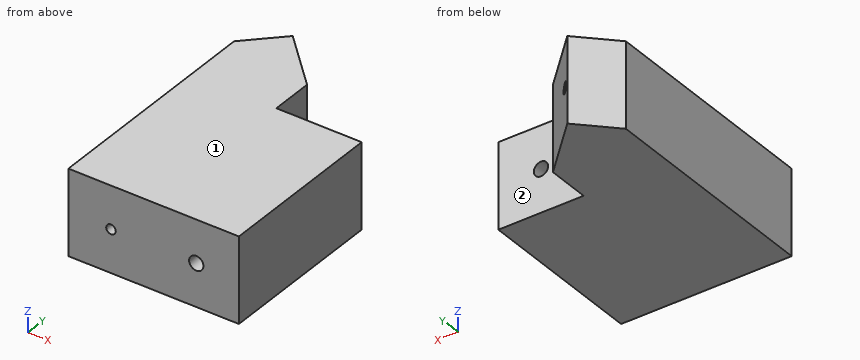
```python
from build123d import *

# Parameters (mm, degrees)
SKETCH1_W               = 10
SKETCH1_H               = 5
BOSS_EXTRUDE1_DEPTH     = 20
SKETCH2_R               = 0.42
SKETCH2_R_2             = 0.28
CUT_EXTRUDE1_DEPTH      = 21
CUT_EXTRUDE2_DEPTH      = 3.5
CUT_EXTRUDE2_DEPTH_BACK = 3.5
CHAMFER1_SIZE2          = 2.828427125
CHAMFER1_SIZE           = 4


with BuildPart() as part:
    # Sketch1 → Boss-Extrude1 (new body)
    with BuildSketch(Plane(origin=(0, 0, 0), x_dir=(1, 0, 0), z_dir=(0, 1, 0))):
        Rectangle(SKETCH1_W, SKETCH1_H)
    extrude(amount=BOSS_EXTRUDE1_DEPTH)

    # Sketch2 → Cut-Extrude1 (cut, through all)
    with BuildSketch(Plane.XZ):
        with Locations((2.5, 0)):
            Circle(SKETCH2_R)
        with Locations((-2.5, 0)):
            Circle(SKETCH2_R_2)
    extrude(amount=-CUT_EXTRUDE1_DEPTH, mode=Mode.SUBTRACT)

    # Sketch3 → Cut-Extrude2 (cut, two sides)
    with BuildSketch(Plane.XY) as cut_extrude2_sk:
        Polygon((-5, 17.5), (0, 12.5), (0, 10), (5, 10), (5, 20), (-5, 20), align=None)
    extrude(amount=CUT_EXTRUDE2_DEPTH, mode=Mode.SUBTRACT)
    extrude(cut_extrude2_sk.sketch, amount=-CUT_EXTRUDE2_DEPTH_BACK, mode=Mode.SUBTRACT)

    # Chamfer1
    chamfer1_edges = [part.edges().sort_by_distance(p)[0] for p in [
        (-5, 17.5, 0),
    ]]
    chamfer(chamfer1_edges, length=CHAMFER1_SIZE, length2=CHAMFER1_SIZE2)


solid = part.part
```
Part model, mm, in its own coordinate system. Face numbers are marked on the shaded views. A direction names the side the tool comes from. Round coordinates to 2 decimals unless told otherwise and drop trailing zeros. Write each loop counter-clockwise with the first axis right and the second up, starting at its lowest first coordinate (ties: lowest second). Pieces come first, ordered by that corner, then holes. Notation, with made-up numbers: M 27,15 L 82,15 A27 ccw 82,54 Z; hole C 85,-1.75 d11. An arc over 180 degrees is marked long. Answer as CSV lines item,"result". Start each with the question number.
1) Drop flat-ended pins along their axis: pin 1 (0.8 mm diameter, centred on y = 12, z = 0, fed in from +X); pin 2 (2.5 mm diameter, centred on x = 2.5, z = 1, fed in from +Y); pin 3 (3 mm diameter, centred on x = -0.5, z = -1.5, fed in from +Y). Give the stop position or say it passes through.
2) Which spindle directions (+Z, -Z, +X, -X, +Y, -Y) get a long thin tool onto all of the face, cutting with end or side? Do the marked faces 1 and 2. Say none if no direction does.
3) Band-saw the part on B-B (z = 0). List the corners of the cut face in (x, y).
4) Band-saw the part on D-D (z = 2.2). List the corners of the cut face in (x, y), then the cut area to 3 significant figures.
5) Drill centre lines: L1, parallel to X at y = 2.5, z = 0; L2, parallel to Z at x = 2.5, y = 3.75; L3, parallel to Z at x = -2.5, y = 10.5. Where is each one in solid material? Low to high.
6) Band-saw the part on A-A (x = -2.5). List the corners of the cut face in (y, z), then the cut area to 3 significant figures.
7) Band-saw the part on C-C (y = 5.5). List the corners of the cut face in (x, z).
Worked out:
1,pin 1,"x = 0"
1,pin 2,"y = 10"
1,pin 3,"y = 14.5"
2,face 1,"+Z, +X, -X, +Y, -Y"
2,face 2,"+Z, -Z, +X, +Y"
3,outline,"M -5,0 L -2.78,0 L -2.78,15.28 L -3,15.5 L -5,13.5 Z; M -2.22,0 L 2.08,0 L 2.08,10 L 0,10 L 0,12.5 L -2.22,14.72 Z; M 2.92,0 L 5,0 L 5,10 L 2.92,10 Z"
4,outline,"M -5,0 L 5,0 L 5,10 L 0,10 L 0,12.5 L -3,15.5 L -5,13.5 Z"
4,area,"121 mm²"
5,L1,"-5 to -2.78, -2.22 to 2.08, 2.92 to 5"
5,L2,"-2.5 to -0.42, 0.42 to 2.5"
5,L3,"-2.5 to -0.28, 0.28 to 2.5"
6,outline,"M 0,-2.5 L 15,-2.5 L 15,-0.28 L 0,-0.28 Z; M 0,0.28 L 15,0.28 L 15,2.5 L 0,2.5 Z"
6,area,"66.6 mm²"
7,outline,"M -5,-2.5 L 5,-2.5 L 5,2.5 L -5,2.5 Z; hole C -2.5,0 d0.56; hole C 2.5,0 d0.84"
